Model file for the job. Use its own axes, mm. Face numbers are marked on the shaded views. A direction names the side the tool comes from. Round coordinates to 2 decimals unless told otherwise and drop trailing zeros. Order: outer loops, then holes, each group sorted by start corner. A loop starts at its lowest first (then second) coordinate and runs counter-clockwise, first axis right, second up. Notation, with made-up numbers: (-0.75, -26.5) -> (37.25, -26.5) arc R13 cw to (37.25, -6.5) -> close; hole circle Ø11 at (27.25, 31.5). An arc over 180 degrees is marked (long way). Use CSV: the item, a comma, the result in double quotes.
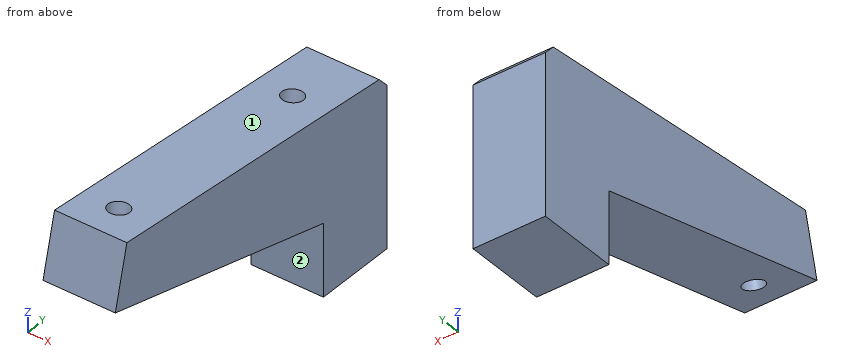
```python
from build123d import *

# Parameters (mm, degrees)
F1_DEPTH = 7
F3_D     = 2
F4_SIZE  = 1


with BuildPart() as f1:
    # F0 (on Right) → F1 (new body)
    with BuildSketch(Plane.YZ):
        Polygon((-26.19513, 6.543331), (0, 0), (0, -7), (8, -7), (8, 9.5), (-24.741056, 12.364471), align=None)
    extrude(amount=F1_DEPTH)

    # F3 (through all)
    with Locations(Plane(origin=(0, 0, 0), x_dir=(1, 0, 0), z_dir=(0, -0.242346, -0.97019))):
        with Locations((3.5, 1.803581), (3.5, 23.5)):
            Hole(F3_D / 2)

    # F4
    f4_edges = [f1.edges().sort_by_distance(p)[0] for p in [
        (3.5, 8, 9.5),
    ]]
    chamfer(f4_edges, length=F4_SIZE)


solid = f1.part
```
Q1. Cut at B-B (x = 5.5). Give the cut face in (y, z), plus the area to 3 significant figures.
From the geometry:
outline,"(-26.2, 6.54) -> (0, 0) -> (0, -7) -> (8, -7) -> (8, 8.5) -> (7, 9.59) -> (-24.74, 12.36) -> close"
area,"341 mm²"
Q2. Cut at A-A (x = 3). Give the cut face in (y, z) (1 decimal), plus the area to 3 significant figures.
From the geometry:
outline,"(-26.2, 6.5) -> (-23.6, 5.9) -> (-22.1, 12.1) -> (-24.7, 12.4) -> close; (-22, 5.5) -> (-2.6, 0.6) -> (-0.2, 10.2) -> (-20.3, 12) -> close; (-0.9, 0.2) -> (0, 0) -> (0, -7) -> (8, -7) -> (8, 8.5) -> (7, 9.6) -> (1.5, 10.1) -> close"
area,"313 mm²"
Q3. Pin check, flat tips, straight feed: pin 1 (8 mm diameter, centred on y = 0.5, z = -3.5, fed in from -X); pin 2 (4 mm diameter, centred on x = 6, y = -6.5, fed in from +Z). Stop position of each tip, or through.
From the geometry:
pin 1,"stops at x = 0"
pin 2,"stops at z = 10.94"
Q4. Probe line 1 along Y through (x, z) = (0.5, -1.25); line 2 along Y through (x, z) = (3.5, 5.5); line 3 along Z through (x, y) = (3.5, -9.5). List the from-to ranges inside material, lowest first.
From the geometry:
line 1,"y = 0 to 8"
line 2,"y = -21.82 to -1.52, 0.55 to 8"
line 3,"z = 2.37 to 11.03"
Q5. Cut at C-C (z = -3.5). Give the cut face in (x, y).
From the geometry:
outline,"(0, 0) -> (7, 0) -> (7, 8) -> (0, 8) -> close"
Q6. Cut at D-D (y = -13). Give the cut face in (x, z), plus the area to 3 significant figures.
From the geometry:
outline,"(0, 3.25) -> (7, 3.25) -> (7, 11.34) -> (0, 11.34) -> close"
area,"56.6 mm²"
Q7. Which spindle directions (+Z, -Z, +X, -X, +Y, -Y) get a long thin tool onto all of the face, cutting with end or side? Do the marked faces 1 and 2. Say none if no direction does.
From the geometry:
face 1,"+Z, +X, -X, +Y"
face 2,"-Z, +X, -X, -Y"
